Study the drawing (mm; zero at the part's minimum x, y, z) and answer. Give positions to 0.01 mm unless a question says otherwise; leave off trailing zeros. Write each loop counter-clockwise with the first axis right and the second up, starting at its lowest first coordinate (ties: lowest second). Pieces come first, ordered by that corner, then holes. Notation, with made-up numbers: (16.5, 57) - (60.5, 57) arc R19 cw to (60.5, 63) - close; hole circle Ø4 at (82.5, 70). An arc over 180 degrees is marked (long way). Write each question's results on one line, items separated by ' | '. Start each with the question number.
Q1. Section A-A (z = 1.2) is taken. Determine the outline of the cut face in (x, y) (3 decimals), plus the area to 3 significant figures.
Q2. Section C-C (x = 140) is taken. Determine the outline of the cut face in (y, z) (3 decimals).
Q3. Section D-D (y = 55.5) is taken. Determine the outline of the cut face in (x, z).
Q4. Section B-B (y = 38.5) is taken. Determine the outline of the cut face in (x, z).
Q5. Find the intervals of material crossed by probe 1 along X at (y, z) = (43, 3.45); probe 2 along Y at (x, z) = (90, 2.9) (3 decimals); probe 3 along X at (y, z) = (49, 2.7), in increasing order.
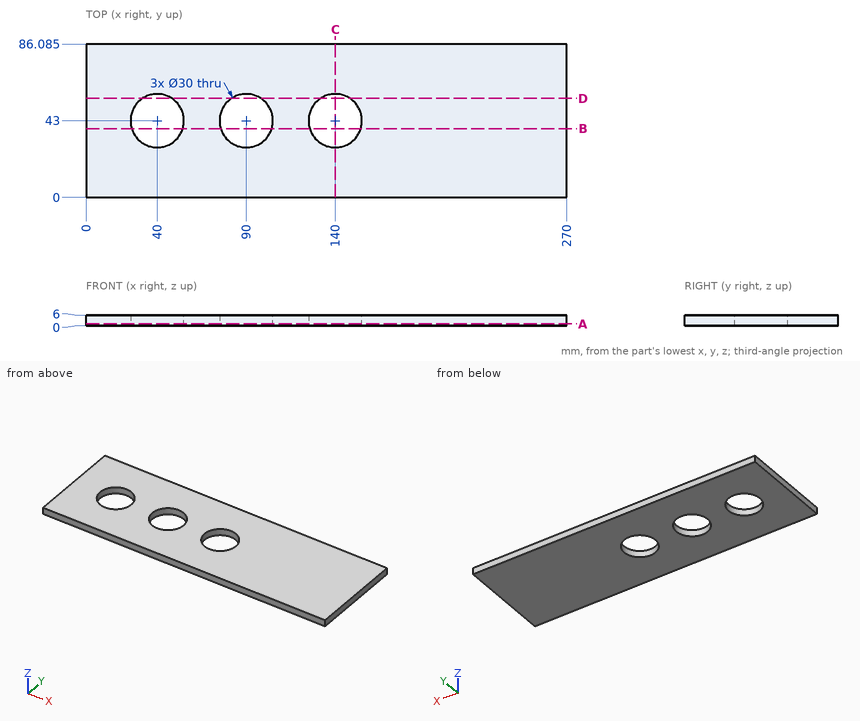
Answers below:
1) outline: (0, 0) - (270, 0) - (270, 86.085) - (0, 86.085) - close; hole circle Ø30 at (40, 43); hole circle Ø30 at (90, 43); hole circle Ø30 at (140, 43) | area: 21,100 mm2
2) outline: (0, 0) - (28, 0) - (28, 6) - (0, 6) - close; (58, 0) - (86.085, 0) - (86.085, 6) - (58, 6) - close
3) outline: (0, 0) - (31.71, 0) - (31.71, 6) - (0, 6) - close; (48.29, 0) - (81.71, 0) - (81.71, 6) - (48.29, 6) - close; (98.29, 0) - (131.71, 0) - (131.71, 6) - (98.29, 6) - close; (148.29, 0) - (270, 0) - (270, 6) - (148.29, 6) - close
4) outline: (0, 0) - (25.69, 0) - (25.69, 6) - (0, 6) - close; (54.31, 0) - (75.69, 0) - (75.69, 6) - (54.31, 6) - close; (104.31, 0) - (125.69, 0) - (125.69, 6) - (104.31, 6) - close; (154.31, 0) - (270, 0) - (270, 6) - (154.31, 6) - close
5) probe 1: x = 0 to 25, 55 to 75, 105 to 125, 155 to 270 | probe 2: y = 0 to 28, 58 to 86.085 | probe 3: x = 0 to 26.25, 53.75 to 76.25, 103.75 to 126.25, 153.75 to 270
